Print and shaded views of the part. All mm, measured from the part's lowest x, y and z. A direction names the side the tool comes from. Give positions to 0.01 mm unless a question says otherwise; leave off trailing zeros. Loops run counter-clockwise (first coordinate to the right, second up) from the corner with the lowest first, then second, coordinate; pieces in that order, holes last. Notation, with made-up numbers: M 50.5,1 L 90.5,1 A20 cw 90.5,26 Z; hole C -29.75,34.5 d4. An arc over 180 degrees is marked long. Answer in a Markdown table with one row per item.
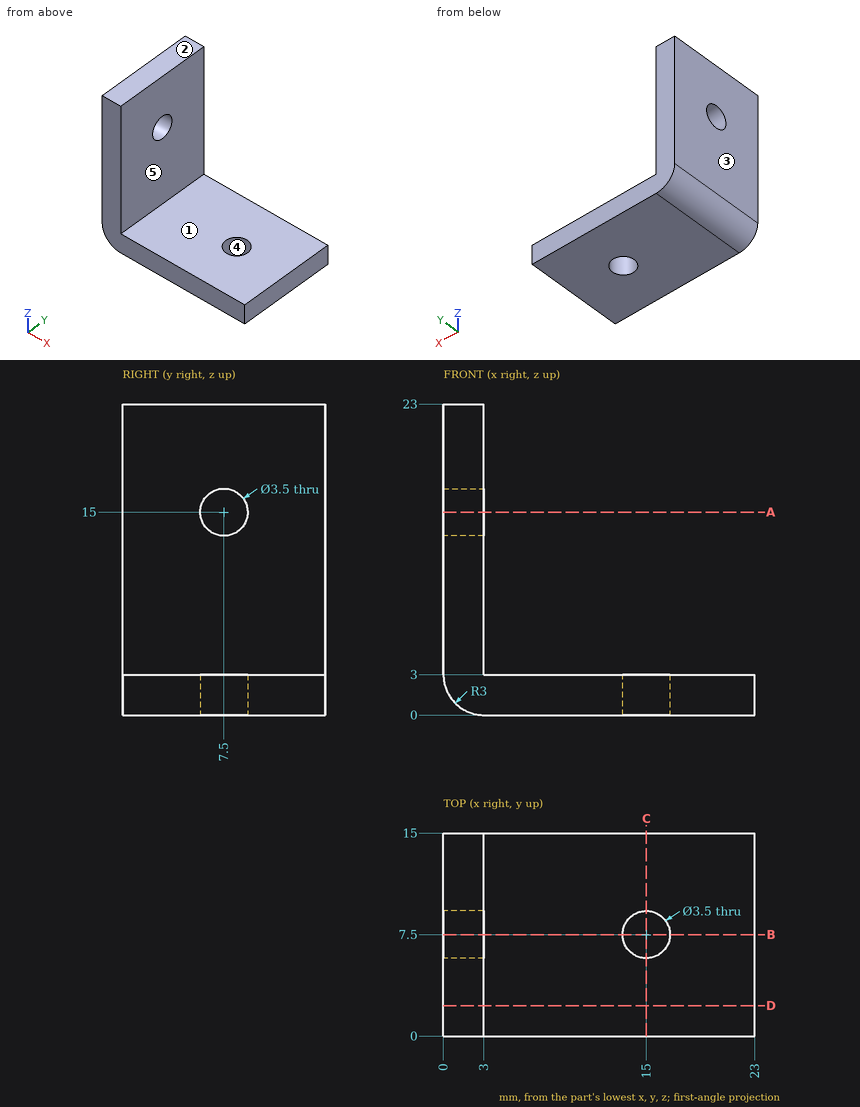
(1) Saw through at B-B, the plane y = 7.5. Give the cut face in (x, z).
Established:
| item | result |
|---|---|
| outline | M 0,3 A3 ccw 3,0 L 13.25,0 L 13.25,3 L 3,3 L 3,13.25 L 0,13.25 Z; M 0,16.75 L 3,16.75 L 3,23 L 0,23 Z; M 16.75,0 L 23,0 L 23,3 L 16.75,3 Z |
(2) Which spindle directions (+Z, -Z, +X, -X, +Y, -Y) get a long thin tool onto all of the face, cutting with end or side? Do the marked faces 1 and 2. Say none if no direction does.
Established:
| item | result |
|---|---|
| face 1 | +Z, +X, +Y, -Y |
| face 2 | +Z, +X, -X, +Y, -Y |
(3) Saw through at C-C, the plane x = 15. Give the cut face in (y, z).
Established:
| item | result |
|---|---|
| outline | M 0,0 L 5.75,0 L 5.75,3 L 0,3 Z; M 9.25,0 L 15,0 L 15,3 L 9.25,3 Z |
(4) Saw through at D-D, the plane y = 2.25. Give the cut face in (x, z).
Established:
| item | result |
|---|---|
| outline | M 0,3 A3 ccw 3,0 L 23,0 L 23,3 L 3,3 L 3,23 L 0,23 Z |
(5) Flat gauge pins, fed straight in: P1, Ø5.5, axis at y = 7.5, z = 15, coming from the +X side; P2, Ø8, axis at x = 17.5, y = 7, coming from the +Z side. Where does each tip first touch, or does it go through?
Established:
| item | result |
|---|---|
| P1 | stops at x = 3 |
| P2 | stops at z = 3 |
(6) Saw through at A-A, the plane z = 15. Give the cut face in (x, y).
Established:
| item | result |
|---|---|
| outline | M 0,0 L 3,0 L 3,5.75 L 0,5.75 Z; M 0,9.25 L 3,9.25 L 3,15 L 0,15 Z |
(7) Mould opens along X. For the marked faces 3, 4 and 5 say: pulls with the +X half, pulls with the -X half, needs draft (parallel to the pull), parting line crosses it, or undercut.
Established:
| item | result |
|---|---|
| face 3 | pulls with the -X half |
| face 4 | undercut |
| face 5 | pulls with the +X half |
(8) Wall check: L1, parallel to Y at x = 1.9, z = 15; L2, parallel to X at y = 6.5, z = 21. Give the ranges that are in metal, low to high.
Established:
| item | result |
|---|---|
| L1 | y = 0 to 5.75, 9.25 to 15 |
| L2 | x = 0 to 3 |
